Verification items for the finished model (mm, model axes). Face numbers are marked on the shaded views. A direction names the side the tool comes from. Coordinates: 2 decimals unless noted, no trailing zeros. Write each loop counter-clockwise with the first axis right and the second up, starting at its lowest first coordinate (ties: lowest second). Pieces come first, ordered by that corner, then holes. Notation, with made-up numbers: M -11,62.5 L 10,62.5 A22 cw 10,73.5 Z; hole C 10.5,-34 d7. An arc over 180 degrees is marked long. Answer in a Markdown table with one row per item.
from build123d import *

# Parameters (mm, degrees)
F2_R = 6
F3_R = 6


with BuildPart() as f1:
    # F0 (on Top) → F1 (revolve)
    with BuildSketch(Plane.XY):
        Polygon((0, 31), (0, 0), (88, 0), (88, 16), (85, 16), (85, 20), (68, 20), (68, 31), align=None)
    revolve(axis=Axis((49.862798, 0, 0), (1, 0, 0)))

    # F2
    f2_edges = [f1.edges().sort_by_distance(p)[0] for p in [
        (0, -31, 0),
    ]]
    fillet(f2_edges, radius=F2_R)

    # F3 (on Top) → F4 (revolve, cut)
    with BuildSketch(Plane.XY):
        with Locations((50, 31)):
            Circle(F3_R)
    revolve(axis=Axis((49.862798, 0, 0), (1, 0, 0)), mode=Mode.SUBTRACT)

    # F5 (on Top) → F6 (revolve, cut)
    with BuildSketch(Plane.XY):
        Polygon((0, 25), (0, 0), (88, 0), (88, 4.04958), (30, 4.04958), (30, 14.04958), (22, 14.04958), (22, 18.54958), (15, 18.54958), (15, 12.5), (12, 12.5), (12, 16), (1.5, 16), (1.5, 25), align=None)
    revolve(axis=Axis((49.862798, 0, 0), (1, 0, 0)), mode=Mode.SUBTRACT)


solid = f1.part
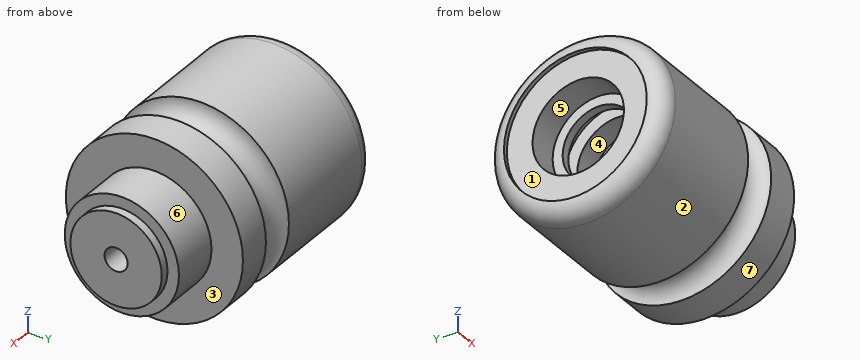
1) Release check for a two-part mould opening along Y. For the marked faces 1, 2 and 3 record: +Y half, -Y half, draft (parallel to the pull), parting line (faces both ways), or undercut.
Response values:
| item | result |
|---|---|
| face 1 | undercut |
| face 2 | parting line |
| face 3 | draft |
2) Thickness scan on L1, parallel to Z at x = 14, y = 0; L2, parallel to X at y = -7.5, z = 16; L3, parallel to X at y = -6.5, z = 14. Record the ranges inside material, lowest first. Write a range as [from, to].
Response values:
| item | result |
|---|---|
| L1 | z = [-31, -12.5], [12.5, 31] |
| L2 | x = [1.5, 15], [22, 85] |
| L3 | x = [12, 15], [22, 88] |
3) Sectioned sample at B-B (x = 45). Record the cut outline in (y, z).
Response values:
| item | result |
|---|---|
| outline | C 0,0 d55.37; hole C 0,0 d8.1 |
4) Tool access check on the marked faces 4, 5, 6 and 7. Record the directions out of +Z, -Z, +X, -X, +Y, -Y that give a thin tool (end or side, any length) a straight path to the whole face; none if there is none.
Response values:
| item | result |
|---|---|
| face 4 | none |
| face 5 | -X |
| face 6 | +X |
| face 7 | +X, -X |
5) Sectioned sample at A-A (x = 63.5). Record the cut outline in (y, z).
Response values:
| item | result |
|---|---|
| outline | C 0,0 d62; hole C 0,0 d8.1 |
6) Depth check by flat-ended pin: pin 1 (15 mm diameter, centred on y = 0, z = 0, fed in from -X); pin 2 (12 mm diameter, centred on x = 29.5, y = -7, fed in from -Z); pin 3 (4 mm diameter, centred on x = 57.5, z = -18.5, fed in from -Y); pin 4 (5 mm diameter, centred on y = 0, z = 0, fed in from +X). Enter the tip coordinate at first touch or a pass-through.
Response values:
| item | result |
|---|---|
| pin 1 | stops at x = 30 |
| pin 2 | stops at z = -30.98 |
| pin 3 | stops at y = -26.24 |
| pin 4 | passes through |
